from build123d import *

# Parameters (mm, degrees)
SKETCH_3_R                = 2.825
CUT_EXTRUDE_2_DEPTH       = 35
SKETCH_14_R               = 1.25
CUT_EXTRUDE_5_DEPTH       = 12
SKETCH_16_W               = 5.008881277
SKETCH_16_H               = 1
EXTRUDE_2_DEPTH           = 30
SKETCH_19_W               = 0.959066555
SKETCH_19_H               = 0.511502163
EXTRUDE_3_DEPTH           = 30
SKETCH_24_W               = 27.218976977
SKETCH_24_H               = 4
CUT_EXTRUDE_8_DEPTH       = 9
SKETCH_25_R               = 1.43
CUT_EXTRUDE_9_DEPTH       = 22
EXTRUDE_4_DEPTH           = 3
EXTRUDE_4_DEPTH_BACK      = 3
CUT_EXTRUDE_12_DEPTH      = 3
CUT_EXTRUDE_12_DEPTH_BACK = 3


with BuildPart() as part:
    # 草圖1 → 旋轉1 (revolve)
    with BuildSketch(Plane.XY, mode=Mode.PRIVATE) as revolve_1_sk:
        Polygon((0, 0), (0, 30), (4, 30), (10, 15.4), (15, 15.4), (21, 30), (25, 30), (25, 15.4), (35, 15.4), (35, 0), align=None)
    revolve(revolve_1_sk.sketch.rotate(Axis((-743.15639781, 0, 0), (1, 0, 0)), 90), axis=Axis((-743.15639781, 0, 0), (1, 0, 0)))

    # 草圖3 → 除料-伸長2 (cut)
    with BuildSketch(Plane(origin=(35, 0, 0), x_dir=(0, 0, -1), z_dir=(1, 0, 0))):
        Circle(SKETCH_3_R)
    extrude(amount=-CUT_EXTRUDE_2_DEPTH, mode=Mode.SUBTRACT)

    # 草圖14 → 除料-伸長5 (cut)
    with BuildSketch(Plane.ZY):
        with Locations((-0.435299539, 17.00388826)):
            Circle(SKETCH_14_R)
    extrude(amount=-CUT_EXTRUDE_5_DEPTH, mode=Mode.SUBTRACT)

    # 草圖16 → 填料-伸長2 (add)
    with BuildSketch(Plane(origin=(35, 0, 0), x_dir=(0, 0, -1), z_dir=(1, 0, 0))):
        with Locations((-0.105543204, 2.350977924)):
            Rectangle(SKETCH_16_W, SKETCH_16_H)
    extrude(amount=-EXTRUDE_2_DEPTH)

    # 草圖19 → 填料-伸長3 (add)
    with BuildSketch(Plane(origin=(35, 0, 0), x_dir=(0, 0, -1), z_dir=(1, 0, 0))):
        with Locations((-0.084116996, 2.673942601)):
            Rectangle(SKETCH_19_W, SKETCH_19_H)
    extrude(amount=-EXTRUDE_3_DEPTH)

    # 草圖24 → 除料-伸長8 (cut)
    with BuildSketch(Plane(origin=(35, 0, 0), x_dir=(0, 0, -1), z_dir=(1, 0, 0))):
        with Locations((1.458428344, 5.180861889)):
            Rectangle(SKETCH_24_W, SKETCH_24_H)
    extrude(amount=-CUT_EXTRUDE_8_DEPTH, mode=Mode.SUBTRACT)

    # 草圖25 → 除料-伸長9 (cut)
    with BuildSketch(Plane(origin=(0, 22, 0), x_dir=(1, 0, 0), z_dir=(0, 1, 0))):
        with Locations(Location((29.956679037, 0, 0), (0, 0, 90))):
            Circle(SKETCH_25_R)
    extrude(amount=-CUT_EXTRUDE_9_DEPTH, mode=Mode.SUBTRACT)

    # 草圖35 → 伸長-薄件4 (add, two sides: drawn at the far end of the back side and taken through both)
    with BuildSketch(Plane.XY.offset(-EXTRUDE_4_DEPTH_BACK)):
        Polygon((17.369423388, -14.9), (7.630576612, -14.9), (12.5, -17.050888526), align=None)
        Polygon((15, -15.4), (10, -15.4), (12.5, -16.504282968), align=None, mode=Mode.SUBTRACT)
    extrude(amount=EXTRUDE_4_DEPTH + EXTRUDE_4_DEPTH_BACK)

    # 草圖36 → 除料-伸長12 (cut, two sides: drawn at the far end of the back side and taken through both)
    with BuildSketch(Plane.XY.offset(-CUT_EXTRUDE_12_DEPTH_BACK)):
        Polygon((11.902920357, -16.787150573), (13.343105155, -16.787150573), (13.343105155, -17.362903865), (11.859661783, -17.362903865), align=None)
    extrude(amount=CUT_EXTRUDE_12_DEPTH + CUT_EXTRUDE_12_DEPTH_BACK, mode=Mode.SUBTRACT)

    # 圓角14
    # a fillet whose section is not a circle: 0.5 mm, written as the material it takes off along each edge
    with BuildSketch(Plane(origin=(11.902920357, -16.787150573, -3.263777256), x_dir=(-0.9147364009889508, 0.4040511313012026, 0), z_dir=(0, 0, 1))) as fillet_14_piece_1:
        with BuildLine():
            add(Edge.make_bspline([(0.105510902, 0), (0.085856889, 0), (0.066202875, 0), (0.022459615, -0.001857581), (-0.01979407, -0.01077403), (-0.060558179, -0.026749346), (-0.078536421, -0.034690573), (-0.096514663, -0.0426318)], knots=[0, 0, 0, 0, 0, 0, 0.5, 0.5, 1, 1, 1, 1, 1, 1], degree=5))
            Line((-0.096514663, -0.0426318), (0, 0))
            Line((0, 0), (0.105510902, 0))
        make_face()
    extrude(amount=6.527554512, mode=Mode.SUBTRACT)
    with BuildSketch(Plane(origin=(13.097079643, -16.787150573, 3.263777256), x_dir=(-1, 0, 0), z_dir=(0, 0, -1))) as fillet_14_piece_2:
        with BuildLine():
            add(Edge.make_bspline([(0.105510902, 0), (0.085856889, 0), (0.066202875, 0), (0.022459615, 0.001857581), (-0.01979407, 0.01077403), (-0.060558179, 0.026749346), (-0.078536421, 0.034690573), (-0.096514663, 0.0426318)], knots=[0, 0, 0, 0, 0, 0, 0.5, 0.5, 1, 1, 1, 1, 1, 1], degree=5))
            Line((-0.096514663, 0.0426318), (0, 0))
            Line((0, 0), (0.105510902, 0))
        make_face()
    extrude(amount=6.527554512, mode=Mode.SUBTRACT)


solid = part.part
The model under review builds one solid part; all positions refer to its coordinate system, in mm. A direction names the side the tool comes from. Round coordinates to 2 decimals unless told otherwise and drop trailing zeros. Write each loop counter-clockwise with the first axis right and the second up, starting at its lowest first coordinate (ties: lowest second). Pieces come first, ordered by that corner, then holes. Notation, with made-up numbers: (59.5, -26) - (115.5, -26) arc R24 cw to (115.5, -4) - close; hole circle Ø3 at (67, 27). An arc over 180 degrees is marked (long way). One line per item, written item: value. Start each with the question number.
1. Consider section A-A on z = 0. State how many separate pieces and enclosed holes the cut face has, and give its area (3 significant figures).
2. To check wall thickness, follow L1, parallel to X at y = 2, z = 0; L2, parallel to X at y = 10.5, z = 0; L3, parallel to Y at x = 33.5, z = -2. State the ranges of each line that lie inside material, in increasing order. Write a range as from..to.
3. Consider section B-B on x = 19.5. Write out the cut boundary in (y, z) (3 decimals), and give its area (3 significant figures).
4. Machinability: for faces 1 (the face through (35, -3, 0)), 2 (the face through (31, 5, 12.151)), 3 (the face through (15.375, -4.9, 15.56)), 4 (the face through (25, -14, -7)), which of the approach directions +Z, -Z, +X, -X, +Y, -Y give a long, thin tool a straight path to every point of the face, cutting with its end or side? Answer none if there is none.
5. The part is to be moulded in two halves that separate along Z. For faces 5 (the face through (20, 1.851, 0)), 6 (the face through (28.54, 2.53, 0.19)), 7 (the face through (32, 7.181, -1)), 8 (the face through (12.535, 15.387, -0.635)), say which applies: released by +Z, released by -Z, zero draft, split by the parting line, or undercut.
6. Clearance check with flat-ended pins moving along their axes: P1, Ø6, axis at x = 23.5, z = -19, coming from the +Y side; P2, Ø2, axis at y = -11, z = -12, coming from the -X side; P3, Ø2.5, axis at x = 29.96, z = 0, coming from the +Y side; P4, Ø5.5, axis at x = 12.5, z = 1.5, coming from the -Y side. State where each tip first meets the part, or that it passes through.
Checks:
1. separate pieces: 5
1. enclosed holes: 1
1. area: 1,240 mm^2
2. L1: x = 5..28.53, 31.39..35
2. L2: x = 0..28.53, 31.39..35
2. L3: y = -15.27..-2, 1.85..3.18, 7.18..15.27
3. outline: circle Ø52.7 at (0, 0); hole (1.851, -2.134) - (1.851, 2.134) arc R2.825 ccw (long way) to start
3. area: 2,160 mm^2
4. face 1: +Z, -Z, +X, +Y, -Y
4. face 2: -Z, +X
4. face 3: none
4. face 4: +X
5. face 5: undercut
5. face 6: undercut
5. face 7: zero draft
5. face 8: split by the parting line
6. P1: stops at y = 25.38
6. P2: stops at x = 0
6. P3: stops at y = -2.53
6. P4: stops at y = -16.79
